Geometry check sheet. Reference: the model listing, model coordinates, mm. Face numbers are marked on the shaded views. A direction names the side the tool comes from. Give positions to 0.01 mm unless a question says otherwise; leave off trailing zeros. Loops run counter-clockwise (first coordinate to the right, second up) from the corner with the lowest first, then second, coordinate; pieces in that order, holes last. Notation, with made-up numbers: (57, 41) -> (84, 41) arc R28 ccw to (84, 65) -> close; hole circle Ø10 at (82.25, 32). An arc over 180 degrees is marked (long way). One line per question, with ' | ' between items.
Autodesk Inventor part; units mm, degrees
ref_plane "SA1_XY" through (0, 0, 0) normal (1, 0, 0) x (0, 0, -1)
ref_plane "SA1_YZ" through (0, 0, 0) normal (0, 0, -1) x (0, 1, 0)
ref_plane "SA1_ZX" through (0, 0, 0) normal (0, 1, 0) x (1, 0, 0)
sketch "Skizze_1" plane through (0, 0, 0) normal (1, 0, 0) x (0, 1, 0)
  line L0 (4.724, 30) -> (1.626, 30)
  line L1 (1.626, 30) -> (1.626, 14.9265)
  arc A0 (1.5502, 14.0803) -> (1.626, 14.9265) centre (-3.134, 14.9265) ccw
  line L2 (1.5502, 14.0803) -> (0.0758, 5.9197)
  arc A1 (0.0758, 5.9197) -> (0, 5.0735) centre (4.76, 5.0735) ccw
  line L3 (0, 5.0735) -> (0, 4.8116)
  arc A2 (-1.389, 2.4058) -> (0, 4.8116) centre (-2.778, 4.8116) ccw
  arc A3 (-1.389, 2.4058) -> (0, -2.778) centre (0, 0) ccw
  line L4 (0, -2.778) -> (6.35, -2.778)
  arc A4 (6.35, -2.778) -> (7.739, 2.4058) centre (6.35, 0) ccw
  arc A5 (6.35, 4.8116) -> (7.739, 2.4058) centre (9.128, 4.8116) ccw
  line L5 (6.35, 4.8116) -> (6.35, 5.0735)
  arc A6 (6.35, 5.0735) -> (6.2742, 5.9197) centre (1.59, 5.0735) ccw
  line L6 (6.2742, 5.9197) -> (4.7998, 14.0803)
  arc A7 (4.724, 14.9265) -> (4.7998, 14.0803) centre (9.484, 14.9265) ccw
  line L7 (4.724, 14.9265) -> (4.724, 30)
extrude "Extrusion1" add sketch "Skizze_1" along normal mid plane 10
sketch "Skizze_2" plane through (0, 0, 0) normal (0, 1, 0) x (-1, 0, 0)
  line L0 (39, 78) -> (-69, 78)
  line L1 (-69, 78) -> (-69, -55)
  line L2 (-69, -55) -> (39, -55)
  line L3 (39, -55) -> (39, 78)
  arc A0 (3.8268, 19.769) -> (0, 27.987) centre (0, 22.987) ccw
  arc A1 (0, 27.987) -> (-3.8268, 19.769) centre (0, 22.987) ccw
  arc A2 (-3.175, 17.9811) -> (-3.8268, 19.769) centre (-5.953, 17.9811) ccw
  line L4 (-3.175, 17.9811) -> (-3.175, 15.2476)
  arc A3 (-3.175, 15.2476) -> (-3.0253, 13.5657) centre (6.35, 15.2476) ccw
  line L5 (-3.0253, 13.5657) -> (-1.6987, 6.1703)
  arc A4 (-1.549, 4.4884) -> (-1.6987, 6.1703) centre (-11.074, 4.4884) ccw
  line L6 (-1.549, 4.4884) -> (-1.549, -2.788)
  line L7 (-1.549, -2.788) -> (1.549, -2.788)
  line L8 (1.549, -2.788) -> (1.549, 4.4884)
  arc A5 (1.6987, 6.1703) -> (1.549, 4.4884) centre (11.074, 4.4884) ccw
  line L9 (1.6987, 6.1703) -> (3.0253, 13.5657)
  arc A6 (3.0253, 13.5657) -> (3.175, 15.2476) centre (-6.35, 15.2476) ccw
  line L10 (3.175, 15.2476) -> (3.175, 17.9811)
  arc A7 (3.8268, 19.769) -> (3.175, 17.9811) centre (5.953, 17.9811) ccw
extrude "Extrusion2" cut sketch "Skizze_2" along normal mid plane 40
sketch "Skizze_3" plane through (0, 0, 0) normal (1, 0, 0) x (0, 1, 0)
  line L0 (10, 22.987) -> (-10, 22.987)
  line L1 (-10, 22.987) -> (-10, 25.137)
  line L2 (-10, 25.137) -> (10, 25.137)
  line L3 (10, 25.137) -> (10, 22.987)
  line L4 (10, 22.987) -> (-10, 22.987)
revolve "Revolution1" cut sketch "Skizze_3" angle 360 about axis through (0, 10, 22.987) along (0, 1, 0)
sketch "Skizze_4" plane through (0, 0, 0) normal (0, 0, 1) x (1, 0, 0)
  line L0 (10, 0) -> (-10, 0)
  line L1 (-10, 0) -> (-10, 1.219)
  line L2 (-10, 1.219) -> (10, 1.219)
  line L3 (10, 1.219) -> (10, 0)
  line L4 (10, 0) -> (-10, 0)
revolve "Revolution2" cut sketch "Skizze_4" angle 360 about axis through (10, 0, 0) along (1, 0, 0)
sketch "Skizze_5" plane through (0, 0, 0) normal (0, 0, 1) x (1, 0, 0)
  line L0 (10, 6.35) -> (-10, 6.35)
  line L1 (-10, 6.35) -> (-10, 7.569)
  line L2 (-10, 7.569) -> (10, 7.569)
  line L3 (10, 7.569) -> (10, 6.35)
  line L4 (10, 6.35) -> (-10, 6.35)
revolve "Revolution3" cut sketch "Skizze_5" angle 360 about axis through (10, 6.35, 0) along (1, 0, 0)
ref_plane "SA1_XY" through (0, 0, 0) normal (1, 0, 0) x (0, 0, -1)
ref_plane "SA1_YZ" through (0, 0, 0) normal (0, 0, -1) x (0, 1, 0)
ref_plane "SA1_ZX" through (0, 0, 0) normal (0, 1, 0) x (1, 0, 0)
ref_plane "SA2_XY" through (0, 6.35, 0) normal (1, 0, 0) x (0, 0, -1)
ref_plane "SA2_YZ" through (0, 6.35, 0) normal (0, 0, -1) x (0, 1, 0)
ref_plane "SA2_ZX" through (0, 6.35, 0) normal (0, 1, 0) x (1, 0, 0)
ref_plane "SA3_XY" through (0, 3.175, 22.987) normal (0, 1, 0) x (1, 0, 0)
ref_plane "SA3_YZ" through (0, 3.175, 22.987) normal (1, 0, 0) x (0, 0, -1)
ref_plane "SA3_ZX" through (0, 3.175, 22.987) normal (0, 0, -1) x (0, 1, 0)
ref_plane "b_left_XY" through (0, 1.626, 27.987) normal (1, 0, 0) x (0, 0, -1)
ref_plane "b_left_YZ" through (0, 1.626, 27.987) normal (0, 0, -1) x (0, 1, 0)
ref_plane "b_left_ZX" through (0, 1.626, 27.987) normal (0, 1, 0) x (1, 0, 0)
ref_plane "r_top_XY" through (0, 9.128, 0) normal (1, 0, 0) x (0, 0, -1)
ref_plane "r_top_YZ" through (0, 9.128, 0) normal (0, 0, -1) x (0, 1, 0)
ref_plane "r_top_ZX" through (0, 9.128, 0) normal (0, 1, 0) x (1, 0, 0)
ref_plane "z_left_XY" through (0, 4.724, 27.987) normal (1, 0, 0) x (0, 0, -1)
ref_plane "z_left_YZ" through (0, 4.724, 27.987) normal (0, 0, -1) x (0, 1, 0)
ref_plane "z_left_ZX" through (0, 4.724, 27.987) normal (0, 1, 0) x (1, 0, 0)
properties part number "205-S-SA"
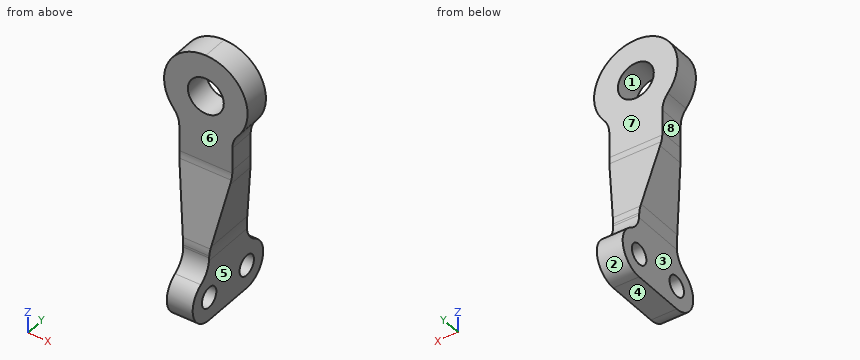
Item 1: Set-up check for the marked faces 4, 5, 6, 7 and 8: record each of +Z, -Z, +X, -X, +Y, -Y from which the full face is reachable in a straight line by a thin tool's end or side.
Result:
face 4: -Z, +X, -X, +Y, -Y | face 5: -Z, +X, +Y, -Y | face 6: +Z, +X, -X, -Y | face 7: +Z, +X, -X, +Y | face 8: -Z, -X, +Y, -Y
Item 2: Release check for a two-part mould opening along Z. For the marked faces 1, 2 and 3 record: pulls with the +Z half, pulls with the -Z half, needs draft (parallel to the pull), parting line crosses it, or undercut.
Result:
face 1: undercut | face 2: parting line crosses it | face 3: needs draft
Item 3: Depth check by flat-ended pin: pin 1 Ø2 at (y, z) = (4, 2.5) entering from -X; pin 2 Ø6 at (y, z) = (3.5, 18) entering from -X; pin 3 Ø0.8 at (y, z) = (3.5, 16) entering from -X (3 decimals); pin 4 Ø4 at (x, y) = (2, 7) entering from -Z. Enter the tip coordinate at first touch or a pass-through.
Result:
pin 1: x = -1.55 | pin 2: x = -4.59 | pin 3: x = -3.175 | pin 4: z = -2.78
Item 4: Scan lines: probe 1 along X at (y, z) = (3.25, 23); probe 2 along Y at (x, z) = (2.25, 22); probe 3 along X at (y, z) = (-2, 0). Record each from-to range of solid material in increasing order.
Result:
probe 1: -5 to -2.15, 2.15 to 5 | probe 2: 1.63 to 4.72 | probe 3: -1.55 to 1.55
Item 5: Sectioned sample at C-C (y = 6.75). Record the cut outline in (x, z), plus the area to 3 significant figures.
Result:
outline: (-1.55, -2.75) -> (1.55, -2.75) -> (1.55, -1.15) -> (-1.55, -1.15) -> close; (-1.55, 1.15) -> (1.55, 1.15) -> (1.55, 3.38) -> (-1.55, 3.38) -> close | area: 11.8 mm2
Item 6: Sectioned sample at A-A (z = 0). Record the cut outline in (x, y), plus the area to 3 significant figures.
Result:
outline: (-1.55, -2.78) -> (1.55, -2.78) -> (1.55, -1.22) -> (-1.55, -1.22) -> close; (-1.55, 1.22) -> (1.55, 1.22) -> (1.55, 5.13) -> (-1.55, 5.13) -> close; (-1.55, 7.57) -> (1.55, 7.57) -> (1.55, 9.13) -> (-1.55, 9.13) -> close | area: 21.8 mm2
Item 7: Sectioned sample at B-B (x = -1). Record the cut outline in (y, z), plus the area to 3 significant figures.
Result:
outline: (-1.39, 2.41) arc R2.78 ccw to (0, -2.78) -> (6.35, -2.78) arc R2.78 ccw to (7.74, 2.41) arc R2.78 cw to (6.35, 4.81) -> (6.35, 5.07) arc R4.76 ccw to (6.27, 5.92) -> (4.8, 14.08) arc R4.76 cw to (4.72, 14.93) -> (4.72, 21.08) -> (1.63, 21.08) -> (1.63, 14.93) arc R4.76 cw to (1.55, 14.08) -> (0.08, 5.92) arc R4.76 ccw to (0, 5.07) -> (0, 4.81) arc R2.78 cw to start; (1.63, 24.89) -> (4.72, 24.89) -> (4.72, 27.89) -> (1.63, 27.89) -> close; hole circle Ø2.44 at (0, 0); hole circle Ø2.44 at (6.35, 0) | area: 141 mm2
Item 8: Sectioned sample at D-D (x = 2.5). Record the cut outline in (y, z).
Result:
outline: (0.93, 10.64) -> (5.42, 10.64) -> (4.8, 14.08) arc R4.76 cw to (4.72, 14.93) -> (4.72, 27.32) -> (1.63, 27.32) -> (1.63, 14.93) arc R4.76 cw to (1.55, 14.08) -> close
